Drawing for the job (mm, zero at the part's lowest x, y, z). Give positions to 0.01 mm unless a question says otherwise; leave off trailing zeros. Write each loop counter-clockwise with the first axis right and the second up, starting at its lowest first coordinate (ties: lowest second). Pieces come first, ordered by that corner, then holes.
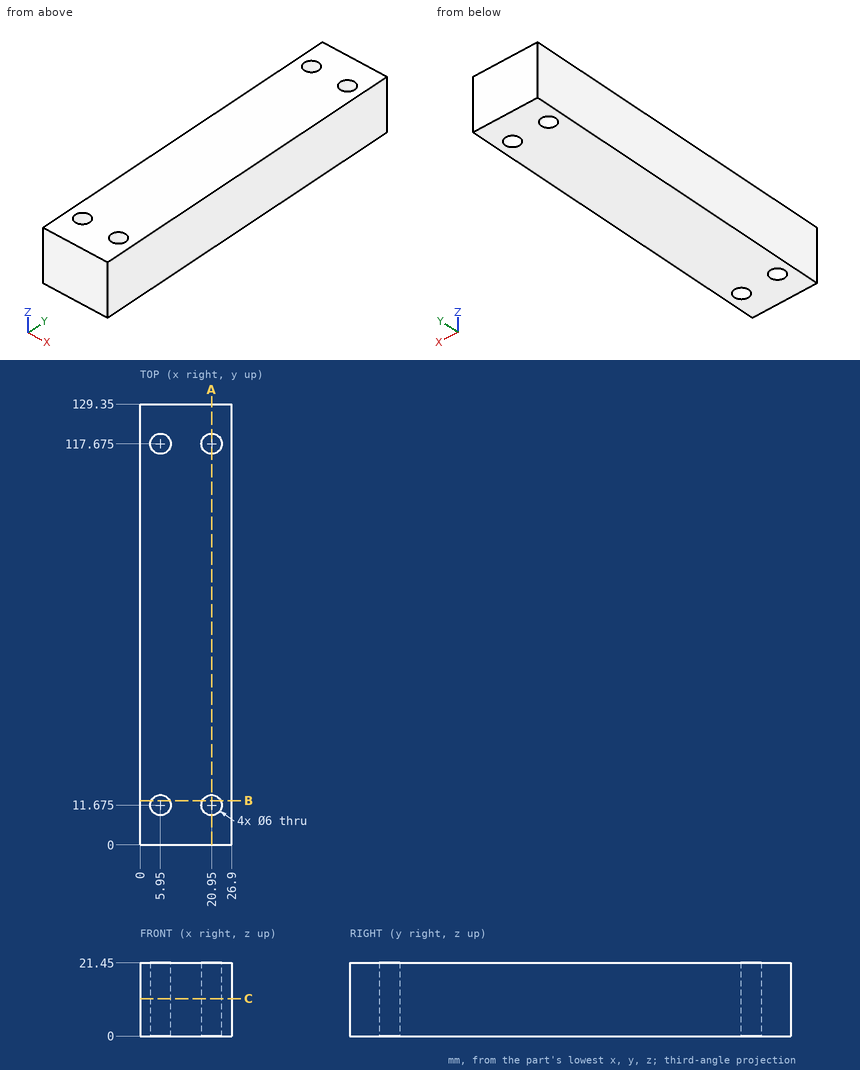
1. Slice it at B-B, the plane y = 13. Write the cut outline in (x, z), and give its area (3 significant figures).
Calculated:
outline: (0, 0) - (3.26, 0) - (3.26, 21.45) - (0, 21.45) - close; (8.64, 0) - (18.26, 0) - (18.26, 21.45) - (8.64, 21.45) - close; (23.64, 0) - (26.9, 0) - (26.9, 21.45) - (23.64, 21.45) - close
area: 346 mm2
2. Slice it at A-A, the plane x = 20.95. Write the cut outline in (y, z) (3 decimals).
Calculated:
outline: (0, 0) - (8.675, 0) - (8.675, 21.45) - (0, 21.45) - close; (14.675, 0) - (114.675, 0) - (114.675, 21.45) - (14.675, 21.45) - close; (120.675, 0) - (129.35, 0) - (129.35, 21.45) - (120.675, 21.45) - close
3. Slice it at C-C, the plane z = 11. Write the cut outline in (x, y) (3 decimals), and give its area (3 significant figures).
Calculated:
outline: (0, 0) - (26.9, 0) - (26.9, 129.35) - (0, 129.35) - close; hole circle Ø6 at (5.95, 11.675); hole circle Ø6 at (5.95, 117.675); hole circle Ø6 at (20.95, 11.675); hole circle Ø6 at (20.95, 117.675)
area: 3,370 mm2
4. Probe probe 1 along Y at (x, z) = (20.95, 7.75) (3 decimals); probe 2 along Y at (x, z) = (3.5, 17.75); probe 3 along X at (y, z) = (117, 9.25). List the from-to ranges inside material, lowest first.
Calculated:
probe 1: y = 0 to 8.675, 14.675 to 114.675, 120.675 to 129.35
probe 2: y = 0 to 9.94, 13.41 to 115.94, 119.41 to 129.35
probe 3: x = 0 to 3.03, 8.87 to 18.03, 23.87 to 26.9
